```python
from build123d import *

# Parameters (mm, degrees)
SKETCH_1_R      = 6
SKETCH_1_R_2    = 2.425
EXTRUDE_1_DEPTH = 0.9
SKETCH_2_R      = 4.5
SKETCH_2_R_2    = 2.425
EXTRUDE_2_DEPTH = 6
FILLET_1_R      = 0.1
CHAMFER_1_SIZE  = 0.4
CHAMFER_1_SIZE2 = 1


with BuildPart() as part:
    # 草图1 → 凸台-拉伸1 (new body)
    with BuildSketch(Plane(origin=(0, 0, 0), x_dir=(1, 0, 0), z_dir=(0, 1, 0))):
        Circle(SKETCH_1_R)
        Circle(SKETCH_1_R_2, mode=Mode.SUBTRACT)
    extrude(amount=EXTRUDE_1_DEPTH)

    # 草图2 → 凸台-拉伸2 (add)
    with BuildSketch(Plane(origin=(0, 0.9, 0), x_dir=(1, 0, 0), z_dir=(0, 1, 0))):
        Circle(SKETCH_2_R)
        Circle(SKETCH_2_R_2, mode=Mode.SUBTRACT)
    extrude(amount=EXTRUDE_2_DEPTH)

    # 圆角1
    fillet_1_edges = [part.edges().sort_by_distance(p)[0] for p in [
        (-2.425, 6.9, 0),
    ]]
    fillet(fillet_1_edges, radius=FILLET_1_R)

    # 倒角1
    chamfer_1_edges = [part.edges().sort_by_distance(p)[0] for p in [
        (-6, 0.9, 0),
    ]]
    chamfer_1_side = [part.faces().sort_by_distance(p)[0] for p in [
        (-6, 0.45, 0),
    ]]
    chamfer(chamfer_1_edges, length=CHAMFER_1_SIZE, length2=CHAMFER_1_SIZE2, reference=chamfer_1_side[0])


solid = part.part
```
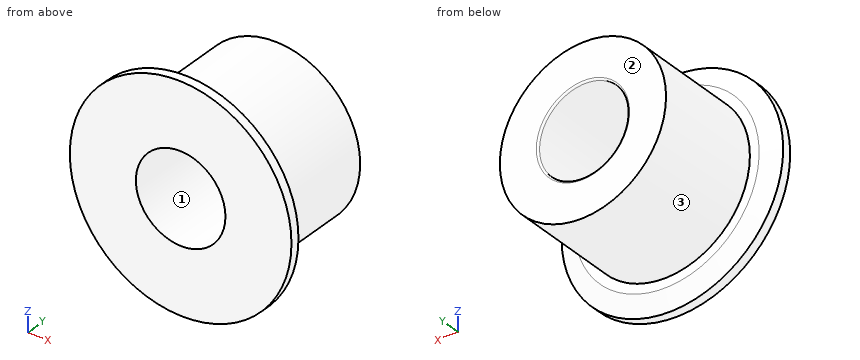
Model file for the job. Use its own axes, mm. Face numbers are marked on the shaded views. Give positions to 0.01 mm unless a question says otherwise; leave off trailing zeros. Write each loop counter-clockwise with the first axis right and the second up, starting at its lowest first coordinate (ties: lowest second). Pieces come first, ordered by that corner, then holes. Notation, with made-up numbers: (57.5, 85) - (89.5, 85) arc R21 ccw to (89.5, 103) - close; hole circle Ø7 at (89.5, 67). An arc over 180 degrees is marked (long way). One line per question, with ' | ' between items. Start each with the question number.
(1) Wall check: line 1 along Z through (x, y) = (0, 3.25) (3 decimals); line 2 along Z through (x, y) = (1.25, 5.25). Give the ranges that are in metal, low to high. Write a range as from..to.
(2) Slice it at C-C on y = 3. Write the cut outline in (x, z) (3 decimals).
(3) Slice it at A-A on z = 0. Write the cut outline in (x, y) (3 decimals).
(4) Slice it at B-B on x = 0. Write the cut outline in (y, z) (3 decimals), plus the area to 3 significant figures.
(5) Two-plate mould, pull along Z, no slides. Class the marked faces 1, 2 and 3: +Z half, -Z half, draft (parallel to the pull), parting line (faces both ways), or undercut.
(6) Pin check, flat tips, straight feed: P1, Ø1, axis at x = 1, z = 0, coming from the +Y side; P2, Ø1, axis at y = 2.5, z = -0.5, coming from the -X side. Stop position of each tip, or through.
Results below:
1) line 1: -4.5..-2.425, 2.425..4.5 | line 2: -4.32..-2.08, 2.08..4.32
2) outline: circle Ø9 at (0, 0); hole circle Ø4.85 at (0, 0)
3) outline: (-6, 0) - (-2.425, 0) - (-2.425, 6.8) arc R0.1 ccw to (-2.525, 6.9) - (-4.5, 6.9) - (-4.5, 0.9) - (-5, 0.9) - (-6, 0.5) - close; (2.425, 0) - (6, 0) - (6, 0.5) - (5, 0.9) - (4.5, 0.9) - (4.5, 6.9) - (2.525, 6.9) arc R0.1 ccw to (2.425, 6.8) - close
4) outline: (0, -6) - (0.5, -6) - (0.9, -5) - (0.9, -4.5) - (6.9, -4.5) - (6.9, -2.525) arc R0.1 ccw to (6.8, -2.425) - (0, -2.425) - close; (0, 2.425) - (6.8, 2.425) arc R0.1 ccw to (6.9, 2.525) - (6.9, 4.5) - (0.9, 4.5) - (0.9, 5) - (0.5, 6) - (0, 6) - close | area: 30.9 mm^2
5) face 1: undercut | face 2: draft | face 3: parting line
6) P1: through | P2: x = -4.5
